Geometry check sheet. Reference: the model listing, model coordinates, mm. Face numbers are marked on the shaded views. A direction names the side the tool comes from. Give positions to 0.01 mm unless a question says otherwise; leave off trailing zeros. Loops run counter-clockwise (first coordinate to the right, second up) from the corner with the lowest first, then second, coordinate; pieces in that order, holes last. Notation, with made-up numbers: (79.25, 66.5) -> (117.25, 66.5) arc R18 cw to (117.25, 73.5) -> close; hole circle Ø10 at (-12, 18). An arc over 180 degrees is marked (long way). Write item = value, one per line.
```python
from build123d import *

# Parameters (mm, degrees)
BOSS_EXTRUDE1_DEPTH = 40
CUT_EXTRUDE1_START  = -40
SKETCH2_R           = 10.8
SKETCH2_R_2         = 5
CUT_EXTRUDE1_DEPTH  = 5
SKETCH2_3_R         = 5
CUT_EXTRUDE2_DEPTH  = 74.759130645
CUT_EXTRUDE3_START  = -40
SKETCH3_R           = 2
CUT_EXTRUDE3_DEPTH  = 15
SKETCH5_R           = 2
CUT_EXTRUDE4_DEPTH  = 72.940583606
FILLET1_R           = 7
SKETCH12_R          = 1.75
CUT_EXTRUDE11_DEPTH = 4
SKETCH14_R          = 3
CUT_EXTRUDE12_DEPTH = 3
SKETCH15_R          = 1.8
CUT_EXTRUDE13_DEPTH = 9
SKETCH16_W          = 40
SKETCH16_H          = 7
BOSS_EXTRUDE5_DEPTH = 2
SKETCH18_W          = 9.7
SKETCH18_H          = 7
BOSS_EXTRUDE6_DEPTH = 4


with BuildPart() as part:
    # Sketch1 → Boss-Extrude1 (new body)
    with BuildSketch(Plane.XY):
        Polygon((-10.843639069, 3.5), (-10.843639069, -3.5), (15.856339325, -3.5), (15.856339325, -39.601683417), (47.6667182, -39.601683417), (47.6667182, -13.398324584), (24.342902039, -13.398324584), (24.342902039, 3.5), align=None)
    extrude(amount=BOSS_EXTRUDE1_DEPTH)

    # Sketch2 → Cut-Extrude1 (cut)
    # profile 1 of 2: a face of its own
    with BuildSketch(Plane.XY.offset(40).offset(CUT_EXTRUDE1_START)):
        with Locations(Location((33.48398225, -26.500004001, 0), (0, 0, 180))):
            Circle(SKETCH2_R)
        with Locations((33.48398225, -26.500004001)):
            Circle(SKETCH2_R_2, mode=Mode.SUBTRACT)
    # profile 2 of 2: a face of its own
    with BuildSketch(Plane.XY.offset(40).offset(CUT_EXTRUDE1_START)):
        with Locations((33.48398225, -26.500004001)):
            Circle(SKETCH2_R_2)
    extrude(amount=CUT_EXTRUDE1_DEPTH, mode=Mode.SUBTRACT)

    # Sketch2<3> → Cut-Extrude2 (cut, through all)
    with BuildSketch(Plane.XY.offset(40)):
        with Locations((33.48398225, -26.500004001)):
            Circle(SKETCH2_3_R)
    extrude(amount=-CUT_EXTRUDE2_DEPTH, mode=Mode.SUBTRACT)

    # Sketch3 → Cut-Extrude3 (cut)
    with BuildSketch(Plane.XY.offset(40).offset(CUT_EXTRUDE3_START)):
        with Locations(Location((33.608608886, -34.499033204, 0), (0, 0, 180))):
            Circle(SKETCH3_R)
        with Locations(Location((25.484953047, -26.624630636, 0), (0, 0, 180))):
            Circle(SKETCH3_R)
        with Locations(Location((33.359355615, -18.500974797, 0), (0, 0, 180))):
            Circle(SKETCH3_R)
        with Locations(Location((41.483011454, -26.375377365, 0), (0, 0, 180))):
            Circle(SKETCH3_R)
    extrude(amount=CUT_EXTRUDE3_DEPTH, mode=Mode.SUBTRACT)

    # Sketch5 → Cut-Extrude4 (cut, through all)
    with BuildSketch(Plane.XZ.offset(3.5)):
        with Locations(Location((-7.343649872, 7.3, 0), (0, 0, 270))):
            Circle(SKETCH5_R)
        with Locations(Location((12.656350128, 7.3, 0), (0, 0, 270))):
            Circle(SKETCH5_R)
        with Locations(Location((-7.343649872, 27.3, 0), (0, 0, 270))):
            Circle(SKETCH5_R)
        with Locations(Location((12.656350128, 27.3, 0), (0, 0, 270))):
            Circle(SKETCH5_R)
    extrude(amount=-CUT_EXTRUDE4_DEPTH, mode=Mode.SUBTRACT)

    # Fillet1
    fillet1_edges = [part.edges().sort_by_distance(p)[0] for p in [
        (24.342902039, 3.5, 20),
        (24.342902039, -13.398324584, 20),
        (47.6667182, -13.398324584, 20),
        (47.6667182, -39.601683417, 20),
        (15.856339325, -39.601683417, 20),
    ]]
    fillet(fillet1_edges, radius=FILLET1_R)

    # Sketch12 → Cut-Extrude11 (cut)
    with BuildSketch(Plane(origin=(0, 0, 0), x_dir=(-1, 0, 0), z_dir=(0, 0, -1))):
        with Locations((-11.169959988, 0)):
            Circle(SKETCH12_R)
        with Locations((7.861665279, 0)):
            Circle(SKETCH12_R)
    extrude(amount=-CUT_EXTRUDE11_DEPTH, mode=Mode.SUBTRACT)

    # Sketch14 → Cut-Extrude12 (cut)
    with BuildSketch(Plane(origin=(0, 3.5, 0), x_dir=(1, 0, 0), z_dir=(0, 1, 0))):
        with Locations(Location((-7.343649872, -7.3, 0), (0, 0, 270))):
            Circle(SKETCH14_R)
        with Locations(Location((-7.343649872, -27.3, 0), (0, 0, 270))):
            Circle(SKETCH14_R)
        with Locations(Location((12.656350128, -27.3, 0), (0, 0, 270))):
            Circle(SKETCH14_R)
        with Locations(Location((12.656350128, -7.3, 0), (0, 0, 270))):
            Circle(SKETCH14_R)
    extrude(amount=-CUT_EXTRUDE12_DEPTH, mode=Mode.SUBTRACT)

    # Sketch15 → Cut-Extrude13 (cut)
    with BuildSketch(Plane.XY.offset(40)):
        with Locations((-7.861665279, 0)):
            Circle(SKETCH15_R)
        with Locations((11.169959988, 0)):
            Circle(SKETCH15_R)
    extrude(amount=-CUT_EXTRUDE13_DEPTH, mode=Mode.SUBTRACT)

    # Sketch16 → Boss-Extrude5 (add)
    with BuildSketch(Plane.ZY.offset(10.843639069)):
        with Locations((20, 0)):
            Rectangle(SKETCH16_W, SKETCH16_H)
    extrude(amount=BOSS_EXTRUDE5_DEPTH)

    # Sketch18 → Boss-Extrude6 (add)
    with BuildSketch(Plane(origin=(0, 0, 0), x_dir=(-1, 0, 0), z_dir=(0, 0, -1))):
        with Locations((-1.506350128, 0)):
            Rectangle(SKETCH18_W, SKETCH18_H)
    boss_extrude6 = extrude(amount=BOSS_EXTRUDE6_DEPTH)

    # Mirror6: Boss-Extrude6 across plane
    add(boss_extrude6.mirror(Plane(origin=(0, 0, 20), x_dir=(1, 0, 0), z_dir=(0, 0, -1))))


solid = part.part
```
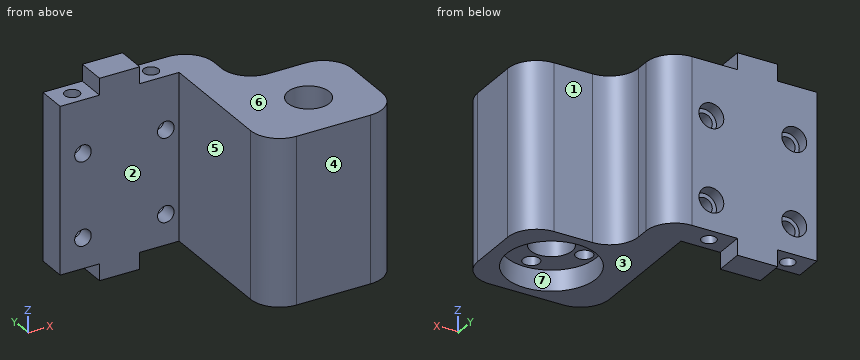
Item 1: Section check D-D, the plane y = -10. Record the cut outline in (x, z).
Answer:
outline = (15.86, 0) -> (25.34, 0) -> (25.34, 40) -> (15.86, 40) -> close
Item 2: Section check B-B, the plane z = 32.5. Record the cut outline in (x, y), plus the area to 3 significant figures.
Answer:
outline = (-12.84, -3.5) -> (15.86, -3.5) -> (15.86, -32.6) arc R7 ccw to (22.86, -39.6) -> (40.67, -39.6) arc R7 ccw to (47.67, -32.6) -> (47.67, -20.4) arc R7 ccw to (40.67, -13.4) -> (31.34, -13.4) arc R7 cw to (24.34, -6.4) -> (24.34, -3.5) arc R7 ccw to (17.34, 3.5) -> (-12.84, 3.5) -> close; hole circle Ø3.6 at (-7.86, 0); hole circle Ø3.6 at (11.17, 0); hole circle Ø10 at (33.48, -26.5)
area = 1,050 mm^2
Item 3: Tool access check on the marked faces 1, 2, 3 and 4. Record the directions out of +Z, -Z, +X, -X, +Y, -Y that give a thin tool (end or side, any length) a straight path to the whole face; none if there is none.
Answer:
face_1 = +Z, -Z, +X, +Y
face_2 = +Z, -Z, -X, -Y
face_3 = -Z, +X, +Y, -Y
face_4 = +Z, -Z, +X, -X, -Y
Item 4: Gauge pin test, flat ends, axial feed: pin 1 (7.5 mm diameter, centred on x = -8, y = -0.5, fed in from -Z); pin 2 (1.8 mm diameter, centred on x = -6.5, z = 26, fed in from +Y); pin 3 (20.5 mm diameter, centred on x = 21.5, y = -24, fed in from +Z). Record the tip position at first contact, or that the pin passes through.
Answer:
pin_1 = 0
pin_2 = 0.5
pin_3 = 40
Item 5: Thickness scan on L1, parallel to Y at x = 33, z = 7.5; L2, parallel to X at y = -2, z = 7; L3, parallel to X at y = -1, z = 7. Record the ranges inside material, lowest first. Write a range as [from, to].
Answer:
L1 = [-39.6, -36.4], [-32.59, -31.48], [-21.52, -20.47], [-16.53, -13.4]
L2 = [-12.84, -9.32], [-5.37, 10.68], [14.63, 24.18]
L3 = [-12.84, -9.32], [-5.37, 10.68], [14.63, 23.88]
Item 6: Draft check along X on the marked faces 5, 6 and 7. Enter one of: +X half, -X half, draft (parallel to the pull), parting line (faces both ways), or undercut.
Answer:
face_5 = -X half
face_6 = draft
face_7 = undercut
Item 7: Section check A-A, the plane z = 27.3. Give the number of separate pieces and of enclosed holes in the cut face, plus the area to 4 significant figures.
Answer:
separate_pieces = 3
enclosed_holes = 1
area = 1,000 mm^2
